Can you work these out from the drawing? Everything is in mm from the part's minimum corner. Round coordinates to 2 decimals unless told otherwise and drop trailing zeros. Loops run counter-clockwise (first coordinate to the right, second up) from the corner with the lowest first, then second, coordinate; pieces in that order, holes last. Notation, with made-up numbers: (8, -35.5) - (20, -35.5) arc R20 cw to (20, -1.5) - close; hole circle Ø11 at (69.25, 18.25). An arc over 180 degrees is marked (long way). Answer as a JSON object with one key per item and string values. Group by question number.
1) If I drill on line 1 along Y through (x, z) = (62.5, 1.8); line 2 along X through (y, z) = (57, 0.5), over which ranges is the centre line in solid material (lowest first)? Write a range as [from, to].
2) I want a section at C-C, the plane x = 81. Please give me the cut outline in (y, z).
3) I want a section at A-A, the plane y = 71. Please give me the cut outline in (x, z), then the cut area to 4 significant figures.
4) I want a section at B-B, the plane z = 1.8. Please give me the cut outline in (x, y).
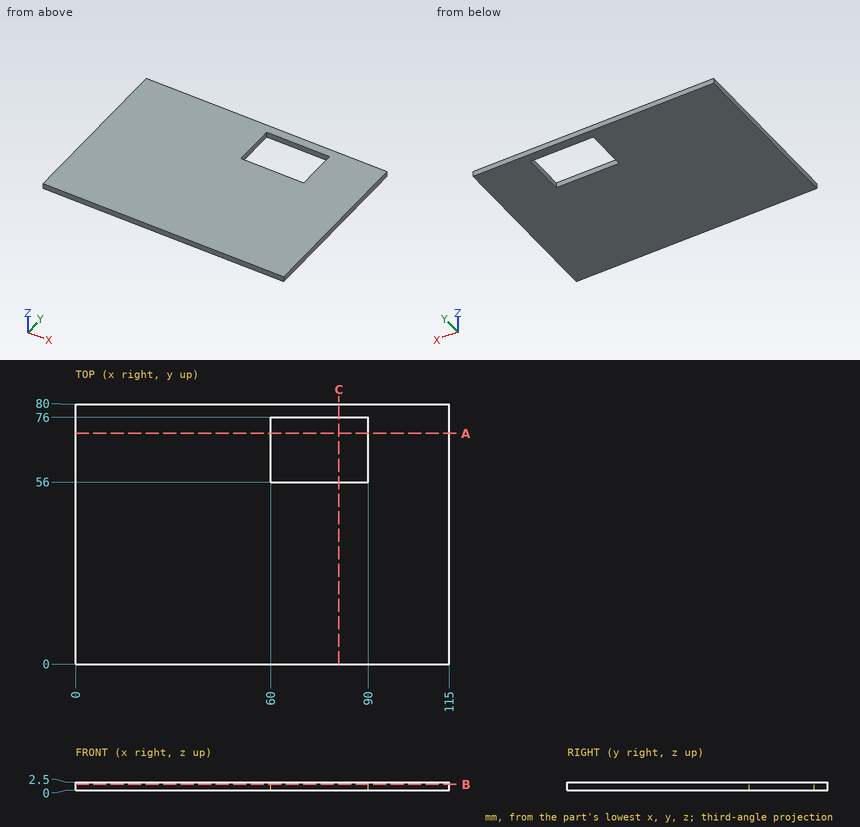
Outcome:
{
 "1": {"line 1": "[0, 56], [76, 80]", "line 2": "[0, 60], [90, 115]"},
 "2": {"outline": "(0, 0) - (56, 0) - (56, 2.5) - (0, 2.5) - close; (76, 0) - (80, 0) - (80, 2.5) - (76, 2.5) - close"},
 "3": {"outline": "(0, 0) - (60, 0) - (60, 2.5) - (0, 2.5) - close; (90, 0) - (115, 0) - (115, 2.5) - (90, 2.5) - close", "area": "212.5 mm^2"},
 "4": {"outline": "(0, 0) - (115, 0) - (115, 80) - (0, 80) - close; hole (60, 56) - (90, 56) - (90, 76) - (60, 76) - close"}
}
